CAD build for the part. Positions are in the model's coordinates, mm. A direction names the side the tool comes from. Coordinates: 2 decimals unless noted, no trailing zeros. Loops run counter-clockwise (first coordinate to the right, second up) from the corner with the lowest first, then second, coordinate; pieces in that order, holes last. Notation, with made-up numbers: (17, -12) -> (25, -12) arc R24 cw to (25, 8) -> close; hole circle Ø6 at (50.5, 27). An arc over 180 degrees is marked (long way). Answer as CSV lines item,"result". Start each with the question number.
from build123d import *

# Parameters (mm, degrees)
SKETCH1_W           = 25
SKETCH1_H           = 17.75
BOSS_EXTRUDE1_DEPTH = 2
BOSS_EXTRUDE2_DEPTH = 3
SKETCH3_W           = 23
SKETCH3_H           = 2
BOSS_EXTRUDE3_DEPTH = 10
CUT_EXTRUDE1_DEPTH  = 8
FILLET1_R           = 1
FILLET2_R           = 0.5
FILLET3_R           = 0.5


with BuildPart() as part:
    # Sketch1 → Boss-Extrude1 (new body)
    with BuildSketch(Plane.XY):
        with Locations((12.5, 8.875)):
            Rectangle(SKETCH1_W, SKETCH1_H)
    extrude(amount=BOSS_EXTRUDE1_DEPTH)

    # Sketch2 → Boss-Extrude2 (add)
    with BuildSketch(Plane.XY.offset(2)):
        Polygon((0, 8.875), (0, 12.375), (4, 12.375), (4, 5.375), (0, 5.375), align=None)
        Polygon((21, 8.875), (21, 12.375), (25, 12.375), (25, 5.375), (21, 5.375), align=None)
    extrude(amount=BOSS_EXTRUDE2_DEPTH)

    # Sketch3 → Boss-Extrude3 (add)
    with BuildSketch(Plane(origin=(0, 0, 0), x_dir=(-1, 0, 0), z_dir=(0, 0, -1))):
        with Locations((-12.5, 2)):
            Rectangle(SKETCH3_W, SKETCH3_H)
    extrude(amount=BOSS_EXTRUDE3_DEPTH)

    # Sketch4 → Cut-Extrude1 (cut)
    with BuildSketch(Plane(origin=(0, 0, -10), x_dir=(-1, 0, 0), z_dir=(0, 0, -1))):
        Polygon((-19.9, 3), (-20.15, 3), (-20.15, 1), (-19.65, 1), (-19.65, 3), align=None)
        Polygon((-22, 3), (-22.25, 3), (-22.25, 1), (-21.75, 1), (-21.75, 3), align=None)
        Polygon((-17.8, 3), (-18.05, 3), (-18.05, 1), (-17.55, 1), (-17.55, 3), align=None)
        Polygon((-15.7, 3), (-15.95, 3), (-15.95, 1), (-15.45, 1), (-15.45, 3), align=None)
        Polygon((-13.6, 3), (-13.85, 3), (-13.85, 1), (-13.35, 1), (-13.35, 3), align=None)
        Polygon((-11.5, 3), (-11.75, 3), (-11.75, 1), (-11.25, 1), (-11.25, 3), align=None)
        Polygon((-9.4, 3), (-9.65, 3), (-9.65, 1), (-9.15, 1), (-9.15, 3), align=None)
        Polygon((-7.3, 3), (-7.55, 3), (-7.55, 1), (-7.05, 1), (-7.05, 3), align=None)
        Polygon((-5.2, 3), (-5.45, 3), (-5.45, 1), (-4.95, 1), (-4.95, 3), align=None)
        Polygon((-3.1, 3), (-3.35, 3), (-3.35, 1), (-2.85, 1), (-2.85, 3), align=None)
    extrude(amount=-CUT_EXTRUDE1_DEPTH, mode=Mode.SUBTRACT)

    # Fillet1
    fillet1_edges = [part.edges().sort_by_distance(p)[0] for p in [
        (0, 0, 1),
        (0, 17.75, 1),
        (25, 17.75, 1),
        (25, 0, 1),
    ]]
    fillet(fillet1_edges, radius=FILLET1_R)

    # Fillet2
    fillet2_edges = [part.edges().sort_by_distance(p)[0] for p in [
        (21.75, 3, -6),
        (22, 1, -2),
        (21.75, 1, -6),
        (22.25, 1, -6),
        (22, 3, -2),
        (22.25, 3, -6),
        (19.65, 3, -6),
        (19.9, 1, -2),
        (19.65, 1, -6),
        (20.15, 1, -6),
        (19.9, 3, -2),
        (20.15, 3, -6),
        (17.55, 3, -6),
        (17.8, 1, -2),
        (17.55, 1, -6),
        (18.05, 1, -6),
        (17.8, 3, -2),
        (18.05, 3, -6),
        (15.45, 3, -6),
        (15.7, 1, -2),
        (15.45, 1, -6),
        (15.95, 1, -6),
        (15.7, 3, -2),
        (15.95, 3, -6),
        (13.35, 3, -6),
        (13.6, 1, -2),
        (13.35, 1, -6),
        (13.85, 1, -6),
        (13.6, 3, -2),
        (13.85, 3, -6),
        (11.25, 3, -6),
        (11.5, 1, -2),
        (11.25, 1, -6),
        (11.75, 1, -6),
        (11.5, 3, -2),
        (11.75, 3, -6),
        (9.15, 3, -6),
        (9.4, 1, -2),
        (9.15, 1, -6),
        (9.65, 1, -6),
        (9.4, 3, -2),
        (9.65, 3, -6),
        (7.05, 3, -6),
        (7.3, 1, -2),
        (7.05, 1, -6),
        (7.55, 1, -6),
        (7.3, 3, -2),
        (7.55, 3, -6),
        (4.95, 3, -6),
        (5.2, 1, -2),
        (4.95, 1, -6),
        (5.45, 1, -6),
        (5.2, 3, -2),
        (5.45, 3, -6),
        (2.85, 3, -6),
        (3.1, 1, -2),
        (2.85, 1, -6),
        (3.35, 1, -6),
        (3.1, 3, -2),
        (3.35, 3, -6),
        (12.5, 1, 0),
        (24, 1, -5),
        (1, 2, 0),
        (1, 1, -5),
        (12.5, 3, 0),
        (1, 3, -5),
        (24, 2, 0),
        (24, 3, -5),
        (23.125, 1, -10),
        (1.925, 3, -10),
        (20.95, 1, -10),
        (18.85, 1, -10),
        (16.75, 1, -10),
        (14.65, 1, -10),
        (12.55, 1, -10),
        (10.45, 1, -10),
        (8.35, 1, -10),
        (6.25, 1, -10),
        (4.15, 1, -10),
        (1.925, 1, -10),
        (4.15, 3, -10),
        (6.25, 3, -10),
        (8.35, 3, -10),
        (10.45, 3, -10),
        (12.55, 3, -10),
        (14.65, 3, -10),
        (16.75, 3, -10),
        (18.85, 3, -10),
        (20.95, 3, -10),
        (23.125, 3, -10),
    ]]
    fillet(fillet2_edges, radius=FILLET2_R)

    # Fillet3
    fillet3_edges = [part.edges().sort_by_distance(p)[0] for p in [
        (2, 5.375, 5),
        (2, 12.375, 5),
        (23, 5.375, 5),
        (23, 12.375, 5),
    ]]
    fillet(fillet3_edges, radius=FILLET3_R)


solid = part.part
Item 1: Saw through at C-C (z = -3.25). Count the separate pieces of the cut face and the enclosed holes in it, plus the area to 3 significant figures.
Item 2: Which spindle directions (+Z, -Z, +X, -X, +Y, -Y) get a long thin tool onto all of the face, cutting with end or side? Do faces 1 (the face through (24, 2, -5)), 2 (the face through (0.285, 17.449, 1.014)), 3 (the face through (19, 2, -10)), 4 (the face through (15.95, 2, -6)), 5 (the face through (23, 5.375, 3)). Say none if no direction does.
Item 3: Saw through at B-B (x = 6.25). Write the cut outline in (y, z).
Item 4: Two-plate mould, pull along X, no slides. Class faces 6 (the face through (0, 9, 2)), 7 (the face through (4.95, 2, -6)), 8 (the face through (10, 2, -10)): pulls with the +X half, pulls with the -X half, needs draft (parallel to the pull), parting line crosses it, or undercut.
Item 5: Flat gauge pins, fed straight in: pin 1 Ø1.5 at (x, y) = (11, 8) entering from -Z; pin 2 Ø0.5 at (y, z) = (2, -6.5) entering from -X; pin 3 Ø0.8 at (y, z) = (2, -5) entering from +X. Where does each tip first touch, or does it go through?
Item 6: Saw through at A-A (y = 8.75). Write the cut outline in (x, z), plus the area to 3 significant figures.
Item 7: Wall check: probe 1 along X at (y, z) = (10.5, 3.5); probe 2 along Y at (x, z) = (15, -7); probe 3 along Z at (x, y) = (11, 14). Give the ranges that are in metal, low to high.
Item 8: Saw through at D-D (y = 13). Write the cut outline in (x, z), plus the area to 3 significant figures.
Geometry check:
1,separate pieces,"11"
1,enclosed holes,"0"
1,area,"33.6 mm2"
2,face 1,"-Z, +X, +Y, -Y"
2,face 2,"+Z, -Z, -X, +Y"
2,face 3,"-Z, +X, -X, +Y, -Y"
2,face 4,"-Z, +Y, -Y"
2,face 5,"+Z, +X, -X, -Y"
3,outline,"(0, 0) -> (0.5, 0) arc R0.5 cw to (1, -0.5) -> (1, -9.5) arc R0.5 ccw to (1.5, -10) -> (2.5, -10) arc R0.5 ccw to (3, -9.5) -> (3, -0.5) arc R0.5 cw to (3.5, 0) -> (17.75, 0) -> (17.75, 2) -> (0, 2) -> close"
4,face 6,"pulls with the -X half"
4,face 7,"undercut"
4,face 8,"needs draft"
5,pin 1,"z = 0"
5,pin 2,"x = 1"
5,pin 3,"x = 24"
6,outline,"(0, 0) -> (25, 0) -> (25, 5) -> (21, 5) -> (21, 2) -> (4, 2) -> (4, 5) -> (0, 5) -> close"
6,area,"74.0 mm2"
7,probe 1,"0 to 4, 21 to 25"
7,probe 2,"1 to 3"
7,probe 3,"0 to 2"
8,outline,"(0, 0) -> (25, 0) -> (25, 2) -> (0, 2) -> close"
8,area,"50.0 mm2"
